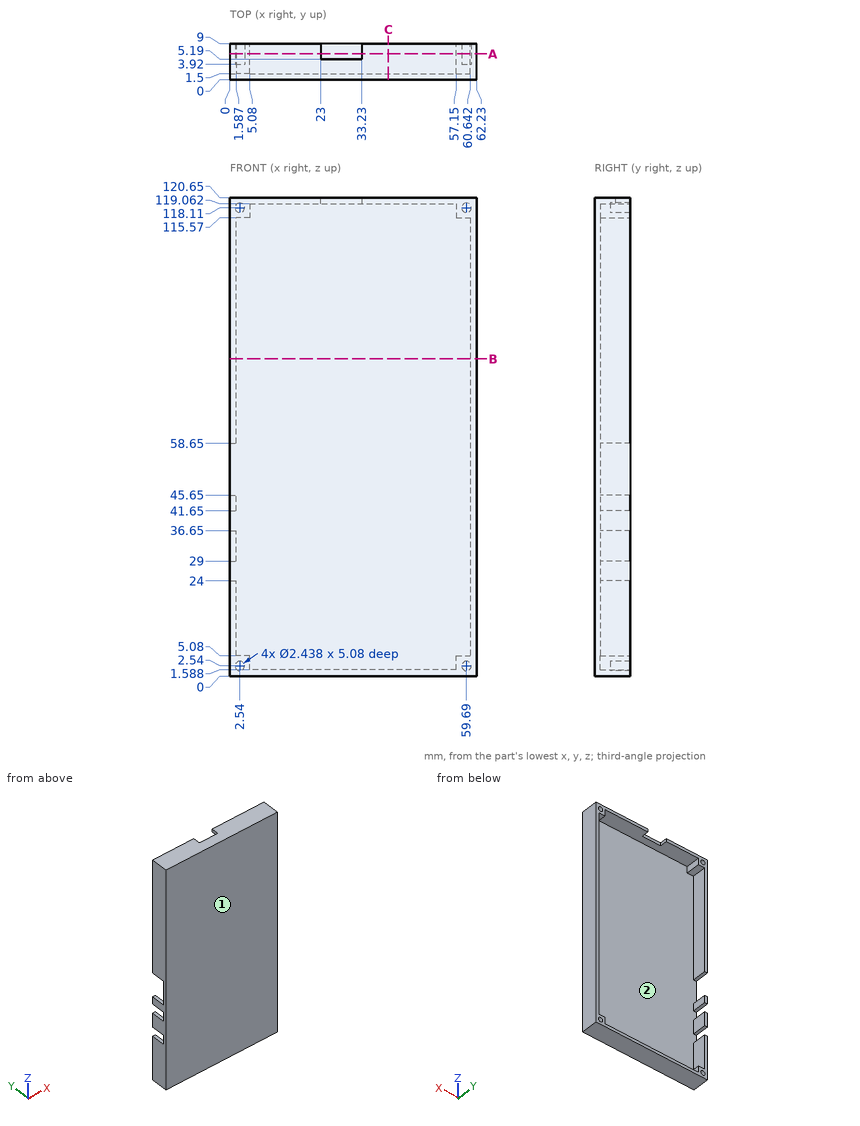
The figure shows three views and two pictorial views of one solid part (mm, origin at its lowest corner). Answer the questions. Round coordinates to 2 decimals unless told otherwise and drop trailing zeros. Loops run counter-clockwise (first coordinate to the right, second up) from the corner with the lowest first, then second, coordinate; pieces in that order, holes last. Notation, with made-up numbers: M 2,50 L 30,50 A22 cw 30,83 Z; hole C 29,69.5 d4. An arc over 180 degrees is marked long. Return JSON: item names as keys, results as strings.
Q1. Find section A-A, the plane y = 6.5. State how many separate pieces and enclosed holes the cut face has.
Results list:
{"separate pieces": "4", "enclosed holes": "4"}
Q2. The mould has two halves that part along Z. Classify the marked faces 1 and 2: released by +Z, released by -Z, zero draft, split by the parting line, or undercut.
Results list:
{"face 1": "zero draft", "face 2": "undercut"}
Q3. Each of these flat-tipped pins is pushed along its axis until it touches: pin 1 Ø1.3 at (x, z) = (28, 119.5) entering from +Y; pin 2 Ø2 at (x, z) = (59.69, 118.11) entering from +Y; pin 3 Ø2 at (x, z) = (33, 40.5) entering from +Y. Where does it stop, or does it pass through?
Results list:
{"pin 1": "stops at y = 5.19", "pin 2": "stops at y = 3.92", "pin 3": "stops at y = 1.5"}
Q4. Find section B-B, the plane z = 80. Determine the outline of the cut face in (x, y), plus the area to 3 significant figures.
Results list:
{"outline": "M 0,0 L 62.23,0 L 62.23,9 L 60.64,9 L 60.64,1.5 L 1.59,1.5 L 1.59,9 L 0,9 Z", "area": "117 mm2"}
Q5. Find section C-C, the plane x = 40. Determine the outline of the cut face in (y, z), plus the area to 3 significant figures.
Results list:
{"outline": "M 0,0 L 9,0 L 9,1.59 L 1.5,1.59 L 1.5,119.06 L 9,119.06 L 9,120.65 L 0,120.65 Z", "area": "205 mm2"}
Q6. Find the intervals of material crossed by line 1 along X through (y, z) = (7.85, 118.11); line 2 along Z through (x, y) = (2.54, 7.65); line 3 along X through (y, z) = (3.75, 8), in increasing order. Write a range as from..to.
Results list:
{"line 1": "x = 0..1.32, 3.76..5.08, 57.15..58.47, 60.91..62.23", "line 2": "z = 0..1.32, 3.76..5.08, 115.57..116.89, 119.33..120.65", "line 3": "x = 0..1.59, 60.64..62.23"}
